For this review, take the finished solid that the model builds, in its own axes (mm). A direction names the side the tool comes from. Round coordinates to 2 decimals unless told otherwise and drop trailing zeros. Order: outer loops, then holes, each group sorted by start corner. A loop starts at its lowest first (then second) coordinate and runs counter-clockwise, first axis right, second up. Notation, with made-up numbers: M 17,-27.75 L 71,-27.75 A23 cw 71,1.25 Z; hole C 57.25,52.25 d11. An arc over 180 degrees is marked long. Write item = value, one per line. Start each with the question number.
from build123d import *

# Parameters (mm, degrees)
SKETCH1_R           = 27
BOSS_EXTRUDE1_DEPTH = 1
BOSS_EXTRUDE3_DEPTH = 2
SKETCH14_R          = 1.5
CUT_EXTRUDE2_DEPTH  = 4
CIRPATTERN2_COUNT   = 4


with BuildPart() as part:
    # Sketch1 → Boss-Extrude1 (new body)
    with BuildSketch(Plane(origin=(0, 0, 0), x_dir=(1, 0, 0), z_dir=(0, 1, 0))):
        Polygon((-31.68, 25.676767512), (-25.68, 31.676767512), (25.68, 31.676767512), (31.68, 25.676767512), (31.68, -25.676767512), (25.68, -31.676767512), (-25.68, -31.676767512), (-31.68, -25.676767512), align=None)
        Circle(SKETCH1_R, mode=Mode.SUBTRACT)
    extrude(amount=BOSS_EXTRUDE1_DEPTH)

    # Sketch2 → Boss-Extrude3 (add)
    with BuildSketch(Plane(origin=(0, 1, 0), x_dir=(1, 0, 0), z_dir=(0, 1, 0))):
        Polygon((26.557063412, 30.799704099), (21.809040421, 26.051681108), (26.051681108, 21.809040421), (30.799704099, 26.557063412), align=None)
        Polygon((30.799704099, -26.557063412), (26.051681108, -21.809040421), (21.809040421, -26.051681108), (26.557063412, -30.799704099), align=None)
        Polygon((-26.557063412, -30.799704099), (-21.809040421, -26.051681108), (-26.051681108, -21.809040421), (-30.799704099, -26.557063412), align=None)
        Polygon((-30.799704099, 26.557063412), (-26.051681108, 21.809040421), (-21.809040421, 26.051681108), (-26.557063412, 30.799704099), align=None)
    extrude(amount=BOSS_EXTRUDE3_DEPTH)

    # Sketch14 → Cut-Extrude2 (cut, through all)
    with BuildSketch(Plane(origin=(0, 3, 0), x_dir=(1, 0, 0), z_dir=(0, 1, 0))):
        with Locations((26.30437226, 26.30437226)):
            Circle(SKETCH14_R)
    cut_extrude2 = extrude(amount=-CUT_EXTRUDE2_DEPTH, mode=Mode.SUBTRACT)

    # CirPattern2: Cut-Extrude2 ×4 about axis
    cirpattern2_axis = Axis((0, 0, 0), (0, 1, 0))
    for i in range(1, CIRPATTERN2_COUNT):
        add(cut_extrude2.rotate(cirpattern2_axis, i * 360 / CIRPATTERN2_COUNT), mode=Mode.SUBTRACT)


solid = part.part
(1) For line 1 along X through (y, z) = (0.6, 0); line 2 along Z through (x, y) = (-26, 1.95); line 3 along X through (y, z) = (1.8, -29), list the stretches that pass through material, from the lowest coordinate up.
(2) We need section A-A, the plane x = 0. Write out the cut boundary in (y, z).
(3) We need section B-B, the plane z = 0. Write out the cut boundary in (x, y), then the cut area to 3 significant figures.
(4) Draft analysis for pull direction X (two halves, no side actions). For faces 4 (the flat face through (-28.722, 1.479, -28.635)), 5 (the flat face through (0, 0, 28)), 6 (the flat face through (0, 1, 28)), state which applies: released by +X, released by -X, zero draft, split by the parting line, or undercut.
(5) For faces 1 (the flat face through (28.39, 1.99, -24.15)), 2 (the flat face through (-28.39, 1.99, 24.15)), 3 (the flat face through (-23.9, 1.99, 23.96)), list the 3-axis set-ups (+Z, -Z, +X, -X, +Y, -Y) from which the entire face can be reached by the end or side of a thin tool; tool diameter is ignored.
(6) We need section C-C, the plane y = 2.4. Write out the cut boundary in (x, z), then the cut area to 3 significant figures.
(7) Insertion check: pin 1 (6 mm diameter, centred on x = 16.5, z = -23.5, fed in from -Y). The pin has a flat end and moves straight along its axis. Give the tip position at first contact, or say it passes through.
Values:
q1.line_1 = -31.68 to -27, 27 to 31.68
q1.line_2 = -30.24 to -27.77, -24.84 to -21.86, 21.86 to 24.84, 27.77 to 30.24
q1.line_3 = -28.36 to -24.76, 24.76 to 28.36
q2.outline = M 0,-31.68 L 1,-31.68 L 1,-27 L 0,-27 Z; M 0,27 L 1,27 L 1,31.68 L 0,31.68 Z
q3.outline = M -31.68,0 L -27,0 L -27,1 L -31.68,1 Z; M 27,0 L 31.68,0 L 31.68,1 L 27,1 Z
q3.area = 9.36 mm²
q4.face_4 = released by -X
q4.face_5 = zero draft
q4.face_6 = undercut
q5.face_1 = +X, +Y
q5.face_2 = -X, +Y
q5.face_3 = +Y
q6.outline = M -30.8,-26.56 L -26.56,-30.8 L -21.81,-26.05 L -26.05,-21.81 Z; M -30.8,26.56 L -26.05,21.81 L -21.81,26.05 L -26.56,30.8 Z; M 21.81,-26.05 L 26.56,-30.8 L 30.8,-26.56 L 26.05,-21.81 Z; M 21.81,26.05 L 26.05,21.81 L 30.8,26.56 L 26.56,30.8 Z; hole C -26.3,-26.3 d3; hole C -26.3,26.3 d3; hole C 26.3,-26.3 d3; hole C 26.3,26.3 d3
q6.area = 133 mm²
q7.pin_1 = 0
